Work out the finished part from the listing and answer in its coordinate system (mm). Face numbers are marked on the shaded views. Round coordinates to 2 decimals unless told otherwise and drop trailing zeros. Loops run counter-clockwise (first coordinate to the right, second up) from the corner with the lowest first, then second, coordinate; pieces in that order, holes last. Notation, with made-up numbers: (-13.75, -14) - (38.25, -14) arc R15 cw to (38.25, 5) - close; hole circle Ø6 at (-21.5, 76.25). An arc over 180 degrees is marked (long way). Use CSV: the item, a comma, the result in double quotes. Start each with the question number.
from build123d import *

# Parameters (mm, degrees)
SKETCH1_W                = 84
SKETCH1_H                = 84
BOSS_EXTRUDE1_DEPTH      = 6
SKETCH2_R                = 1.5
CUT_EXTRUDE1_DEPTH       = 119.94536561
CUT_EXTRUDE2_DEPTH       = 119.94536561
CIRPATTERN1_COUNT        = 3
CIRPATTERN1_ANGLE        = 180
CIRPATTERN1_COPY_1_DEPTH = 119.94536561
CIRPATTERN1_COPY_2_DEPTH = 119.94536561
SKETCH4_R                = 1.5
CUT_EXTRUDE4_DEPTH       = 3
MIRROR3_COPY_1_SKETCH_R  = 1.5
MIRROR3_COPY_1_DEPTH     = 3


with BuildPart() as part:
    # Sketch1 → Boss-Extrude1 (new body)
    with BuildSketch(Plane(origin=(0, 0, 0), x_dir=(1, 0, 0), z_dir=(0, 1, 0))):
        with Locations((42, 42)):
            Rectangle(SKETCH1_W, SKETCH1_H)
    extrude(amount=BOSS_EXTRUDE1_DEPTH)

    # Sketch2 → Cut-Extrude1 (cut, through all)
    with BuildSketch(Plane(origin=(0, 6, 0), x_dir=(1, 0, 0), z_dir=(0, 1, 0))):
        with Locations(Location((6, 72, 0), (0, 0, 270))):
            Circle(SKETCH2_R)
        with Locations(Location((6, 12, 0), (0, 0, 270))):
            Circle(SKETCH2_R)
        with Locations(Location((78, 12, 0), (0, 0, 270))):
            Circle(SKETCH2_R)
        with Locations(Location((78, 72, 0), (0, 0, 270))):
            Circle(SKETCH2_R)
    extrude(amount=-CUT_EXTRUDE1_DEPTH, mode=Mode.SUBTRACT)

    # Sketch3 → Cut-Extrude2 (cut, through all)
    with BuildSketch(Plane(origin=(0, 6, 0), x_dir=(1, 0, 0), z_dir=(0, 1, 0))):
        Polygon((24.5, 76), (59.5, 76), (59.5, 70.813708499), (42, 53.313708499), (24.5, 70.813708499), align=None)
    cut_extrude2 = extrude(amount=-CUT_EXTRUDE2_DEPTH, mode=Mode.SUBTRACT)

    # Mirror1: Cut-Extrude2 across plane
    add(cut_extrude2.mirror(Plane.XY.offset(-42)), mode=Mode.SUBTRACT)

    # CirPattern1: Cut-Extrude2 ×3 about axis
    cirpattern1_axis = Axis((42, 0, -42), (0, 1, 0))
    for i in range(1, CIRPATTERN1_COUNT):
        add(cut_extrude2.rotate(cirpattern1_axis, i * CIRPATTERN1_ANGLE / (CIRPATTERN1_COUNT - 1)), mode=Mode.SUBTRACT)

    # CirPattern1 copy 1 sketch → CirPattern1 copy 1 (cut, through all)
    with BuildSketch(Plane(origin=(0, 6, 0), x_dir=(0, 0, -1), z_dir=(0, 1, 0))):
        Polygon((24.5, -76), (59.5, -76), (59.5, -70.813708499), (42, -53.313708499), (24.5, -70.813708499), align=None)
    extrude(amount=-CIRPATTERN1_COPY_1_DEPTH, mode=Mode.SUBTRACT)

    # CirPattern1 copy 2 sketch → CirPattern1 copy 2 (cut, through all)
    with BuildSketch(Plane(origin=(84, 6, 0), x_dir=(-1, 0, 0), z_dir=(0, 1, 0))):
        Polygon((24.5, -76), (59.5, -76), (59.5, -70.813708499), (42, -53.313708499), (24.5, -70.813708499), align=None)
    extrude(amount=-CIRPATTERN1_COPY_2_DEPTH, mode=Mode.SUBTRACT)

    # Sketch4 → Cut-Extrude4 (cut)
    with BuildSketch(Plane(origin=(0, 6, 0), x_dir=(1, 0, 0), z_dir=(0, 1, 0))):
        Polygon((14, 14), (14, 8), (2, 8), (2, 20), (8, 20), align=None)
        with Locations(Location((6, 12, 0), (0, 0, 270))):
            Circle(SKETCH4_R, mode=Mode.SUBTRACT)
    cut_extrude4 = extrude(amount=-CUT_EXTRUDE4_DEPTH, mode=Mode.SUBTRACT)

    # Mirror2: Cut-Extrude4 across plane
    add(cut_extrude4.mirror(Plane.XY.offset(-42)), mode=Mode.SUBTRACT)

    # Mirror3: Cut-Extrude4 across plane
    add(cut_extrude4.mirror(Plane.ZY.offset(-42)), mode=Mode.SUBTRACT)

    # Mirror3 copy 1 sketch → Mirror3 copy 1 (cut)
    with BuildSketch(Plane(origin=(84, 6, -84), x_dir=(-1, 0, 0), z_dir=(0, 1, 0))):
        Polygon((14, 14), (14, 8), (2, 8), (2, 20), (8, 20), align=None)
        with Locations(Location((6, 12, 0), (0, 0, 270))):
            Circle(MIRROR3_COPY_1_SKETCH_R, mode=Mode.SUBTRACT)
    extrude(amount=-MIRROR3_COPY_1_DEPTH, mode=Mode.SUBTRACT)


solid = part.part
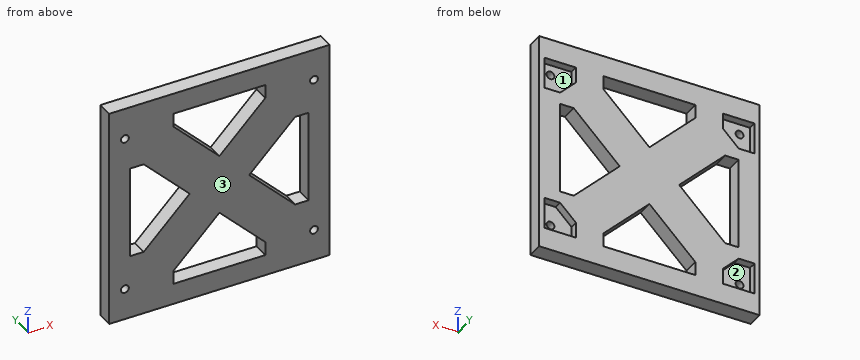
Item 1: A cutting plane is placed at A-A (z = -12). Determine the outline of the cut face in (x, y), plus the area to 3 significant figures.
Item 2: A cutting plane is placed at B-B (x = 6). Determine the outline of the cut face in (y, z).
Item 3: A cutting plane is placed at D-D (z = -32.5). Determine the outline of the cut face in (x, y).
Item 4: The mould has two halves that part along Z. Classify the marked faces 1, 2 and 3: pulls with the +Z half, pulls with the -Z half, needs draft (parallel to the pull), parting line crosses it, or undercut.
Item 5: Find the intervals of material crossed by probe 1 along Z at (x, y) = (78, 1.5); probe 2 along X at (y, z) = (3.75, -9); probe 3 along X at (y, z) = (1.05, -72), in increasing order. Write a range as [from, to].
Item 6: A cutting plane is placed at C-C (x = 26.5). Determine the outline of the cut face in (y, z), plus the area to 3 significant figures.
Item 7: Each of these flat-tipped pins is pushed along its axis until it touches: pin 1 Ø1.5 at (y, z) = (3, -67.5) entering from -X; pin 2 Ø6 at (x, z) = (7.5, -68) entering from +Y. Where does it stop, or does it pass through?
Result sheet:
1,outline,"(0, 0) - (4.5, 0) - (4.5, 3) - (2, 3) - (2, 6) - (0, 6) - close; (7.5, 0) - (24.5, 0) - (24.5, 6) - (14, 6) - (14, 3) - (7.5, 3) - close; (59.5, 0) - (76.5, 0) - (76.5, 3) - (70, 3) - (70, 6) - (59.5, 6) - close; (79.5, 0) - (84, 0) - (84, 6) - (82, 6) - (82, 3) - (79.5, 3) - close"
1,area,"204 mm^2"
2,outline,"(0, -84) - (6, -84) - (6, -76) - (3, -76) - (3, -73.5) - (0, -73.5) - close; (0, -70.5) - (3, -70.5) - (3, -64) - (6, -64) - (6, -20) - (3, -20) - (3, -13.5) - (0, -13.5) - close; (0, -10.5) - (3, -10.5) - (3, -8) - (6, -8) - (6, 0) - (0, 0) - close"
3,outline,"(0, 0) - (8, 0) - (8, 6) - (0, 6) - close; (21.19, 0) - (62.81, 0) - (62.81, 6) - (21.19, 6) - close; (76, 0) - (84, 0) - (84, 6) - (76, 6) - close"
4,face 1,"undercut"
4,face 2,"undercut"
4,face 3,"needs draft"
5,probe 1,"[-84, -73.5], [-70.5, -13.5], [-10.5, 0]"
5,probe 2,"[0, 2], [14, 24.5], [59.5, 70], [82, 84]"
5,probe 3,"[0, 4.5], [7.5, 24.5], [59.5, 76.5], [79.5, 84]"
6,outline,"(0, -84) - (6, -84) - (6, -76) - (0, -76) - close; (0, -68.81) - (6, -68.81) - (6, -46.19) - (0, -46.19) - close; (0, -37.81) - (6, -37.81) - (6, -15.19) - (0, -15.19) - close; (0, -8) - (6, -8) - (6, 0) - (0, 0) - close"
6,area,"368 mm^2"
7,pin 1,"x = 0"
7,pin 2,"y = 3"
